Autodesk Fusion 360 part; units mm, degrees
sketch "baseplate" plane through (0, 0, 0) normal (0, 1, 0) x (1, 0, 0)
  line L0 (0, 0) -> (80, 0)
  line L1 (80, 0) -> (80, -40)
  line L2 (80, -40) -> (0, -40)
  line L3 (0, -40) -> (0, 0)
  dimension "d1" = 80
  dimension "d2" = 40
sketch "pryamid_base" plane through (0, 0, 0) normal (0, 1, 0) x (1, 0, 0)
  line L0 (5, -35) -> (15, -35)
  line L1 (15, -35) -> (15, -25)
  line L2 (15, -25) -> (5, -25)
  line L3 (5, -25) -> (5, -35)
  line L4 (35, -35) -> (35, -25)
  line L5 (35, -25) -> (25, -25)
  line L6 (25, -35) -> (35, -35)
  line L7 (25, -25) -> (25, -35)
  line L8 (75, -35) -> (75, -25)
  line L9 (45, -35) -> (55, -35)
  line L10 (55, -25) -> (45, -25)
  line L11 (65, -25) -> (65, -35)
  line L12 (65, -35) -> (75, -35)
  line L13 (55, -35) -> (55, -25)
  line L14 (45, -25) -> (45, -35)
  line L15 (75, -25) -> (65, -25)
  line L16 (35, -5) -> (25, -5)
  line L17 (35, -15) -> (35, -5)
  line L18 (15, -5) -> (5, -5)
  line L19 (25, -5) -> (25, -15)
  line L20 (45, -15) -> (55, -15)
  line L21 (55, -15) -> (55, -5)
  line L22 (5, -5) -> (5, -15)
  line L23 (45, -5) -> (45, -15)
  line L24 (75, -15) -> (75, -5)
  line L25 (65, -5) -> (65, -15)
  line L26 (75, -5) -> (65, -5)
  line L27 (55, -5) -> (45, -5)
  line L28 (65, -15) -> (75, -15)
  line L29 (5, -15) -> (15, -15)
  line L30 (15, -15) -> (15, -5)
  line L31 (25, -15) -> (35, -15)
  dimension "d3" = 10
  dimension "d4" = 10
  dimension "d5" = 10
  dimension "d6" = 10
  dimension "d7" = 10
  dimension "d8" = 10
  dimension "d9" = 10
  dimension "d10" = 10
  dimension "d11" = 10
  dimension "d12" = 10
  dimension "d13" = 10
  dimension "d14" = 10
  dimension "d15" = 10
  dimension "d16" = 10
  dimension "d17" = 10
  dimension "d18" = 10
ref_plane "WorkPlane1" through (0, 4.5, 0) normal (0, 1, 0) x (0, 0, 1)
sketch "pryamid_offsetplane" plane through (0, 4.5, 0) normal (0, 1, 0) x (1, 0, 0)
  line L0 (7.5, -32.5) -> (12.5, -32.5)
  line L1 (12.5, -32.5) -> (12.5, -27.5)
  line L2 (12.5, -27.5) -> (7.5, -27.5)
  line L3 (7.5, -27.5) -> (7.5, -32.5)
  line L4 (27.5, -27.5) -> (27.5, -32.5)
  line L5 (32.5, -32.5) -> (32.5, -27.5)
  line L6 (27.5, -32.5) -> (32.5, -32.5)
  line L7 (32.5, -27.5) -> (27.5, -27.5)
  line L8 (7.5, -27.5) -> (7.5, -32.5)
  line L9 (12.5, -32.5) -> (12.5, -27.5)
  line L10 (7.5, -32.5) -> (12.5, -32.5)
  line L11 (12.5, -27.5) -> (7.5, -27.5)
  line L12 (47.5, -27.5) -> (47.5, -32.5)
  line L13 (52.5, -32.5) -> (52.5, -27.5)
  line L14 (47.5, -32.5) -> (52.5, -32.5)
  line L15 (52.5, -27.5) -> (47.5, -27.5)
  line L16 (67.5, -27.5) -> (67.5, -32.5)
  line L17 (72.5, -32.5) -> (72.5, -27.5)
  line L18 (67.5, -32.5) -> (72.5, -32.5)
  line L19 (72.5, -27.5) -> (67.5, -27.5)
  line L20 (72.5, -12.5) -> (72.5, -7.5)
  line L21 (27.5, -7.5) -> (27.5, -12.5)
  line L22 (12.5, -12.5) -> (12.5, -7.5)
  line L23 (72.5, -7.5) -> (67.5, -7.5)
  line L24 (12.5, -7.5) -> (7.5, -7.5)
  line L25 (52.5, -12.5) -> (52.5, -7.5)
  line L26 (7.5, -7.5) -> (7.5, -12.5)
  line L27 (7.5, -12.5) -> (12.5, -12.5)
  line L28 (47.5, -12.5) -> (52.5, -12.5)
  line L29 (67.5, -7.5) -> (67.5, -12.5)
  line L30 (47.5, -7.5) -> (47.5, -12.5)
  line L31 (67.5, -12.5) -> (72.5, -12.5)
  line L32 (32.5, -7.5) -> (27.5, -7.5)
  line L33 (52.5, -7.5) -> (47.5, -7.5)
  line L34 (27.5, -12.5) -> (32.5, -12.5)
  line L35 (12.5, -7.5) -> (7.5, -7.5)
  line L36 (32.5, -12.5) -> (32.5, -7.5)
  line L37 (12.5, -12.5) -> (12.5, -7.5)
  line L38 (7.5, -12.5) -> (12.5, -12.5)
  line L39 (7.5, -7.5) -> (7.5, -12.5)
extrude "Extrude1" add sketch "baseplate" against normal blind 5
loft "Loft1" add profiles "pryamid_base", "pryamid_offsetplane" section 1 contours L0 L1 L2 L3 section 2 contours L0 L1 L2 L3 L8 L9 L10 L11
loft "Loft2" add profiles "pryamid_base", "pryamid_offsetplane" section 1 contours L4 L5 L6 L7 section 2 contours L4 L5 L6 L7
loft "Loft3" add profiles "pryamid_base", "pryamid_offsetplane" section 1 contours L9 L10 L13 L14 section 2 contours L12 L13 L14 L15
loft "Loft4" add profiles "pryamid_base", "pryamid_offsetplane" section 1 contours L8 L11 L12 L15 section 2 contours L16 L17 L18 L19
loft "Loft5" add profiles "pryamid_base", "pryamid_offsetplane" section 1 contours L24 L25 L26 L28 section 2 contours L20 L23 L29 L31
loft "Loft6" add profiles "pryamid_base", "pryamid_offsetplane" section 1 contours L20 L21 L23 L27 section 2 contours L25 L28 L30 L33
loft "Loft7" add profiles "pryamid_base", "pryamid_offsetplane" section 1 contours L16 L17 L19 L31 section 2 contours L21 L32 L34 L36
loft "Loft8" add profiles "pryamid_base", "pryamid_offsetplane" section 1 contours L18 L22 L29 L30 section 2 contours L22 L24 L26 L27 L35 L37 L38 L39
sketch "sidewall" plane through (0, 0, 0) normal (0, 1, 0) x (1, 0, 0)
  line L0 (0, 0) -> (-8, 0)
  line L1 (-8, 0) -> (-8, -40)
  line L2 (-8, -40) -> (0, -40)
  line L3 (0, -40) -> (0, 0)
  dimension "d22" = 8
extrude "Extrude2" add sketch "sidewall" along normal blind 0 and the other way blind 5
sketch "sidemount" plane through (0, 0, 0) normal (0, 1, 0) x (1, 0, 0)
  line L0 (80, 0) -> (88, 0)
  line L1 (88, 0) -> (88, -40)
  line L2 (88, -40) -> (80, -40)
  line L3 (80, -40) -> (80, 0)
extrude "Extrude3" add sketch "sidemount" against normal blind 5
sketch "holes" plane through (0, -5, 0) normal (0, -1, 0) x (1, 0, 0)
  line L0 (88, 40) -> (-8, 40)
  line L1 (-8, 40) -> (-8, 0)
  line L2 (-8, 0) -> (88, 0)
  line L3 (88, 0) -> (88, 40)
  line L4 (-8, 0) -> (-4, 0)
  line L5 (-8, 6) -> (-8, 0)
  line L6 (-4, 40) -> (-8, 40)
  line L7 (-8, 40) -> (-8, 34)
  circle A0 centre (-4, 34) radius 2
  circle A1 centre (-4, 6) radius 2
  circle A2 centre (-4, 34) radius 3.4
  circle A3 centre (-4, 6) radius 3.4
  dimension "d29" = 6
  dimension "d30" = 4
  dimension "d31" = 4
  dimension "d32" = 6.8
  dimension "d33" = 6.8
extrude "Extrude4" cut sketch "holes" against normal blind 51 contours A0 | A1
sketch "Sketch7" plane through (0, -5, 0) normal (0, -1, 0) x (1, 0, 0)
  circle A0 centre (84, 34) radius 2
  circle A1 centre (84, 6) radius 2
  circle A2 centre (84, 34) radius 3.4
  circle A3 centre (84, 6) radius 3.4
  dimension "d42" = 4
  dimension "d43" = 4
  dimension "d44" = 6.8
  dimension "d45" = 6.8
extrude "Extrude6" cut sketch "Sketch7" against normal blind 16 contours A0 | A1
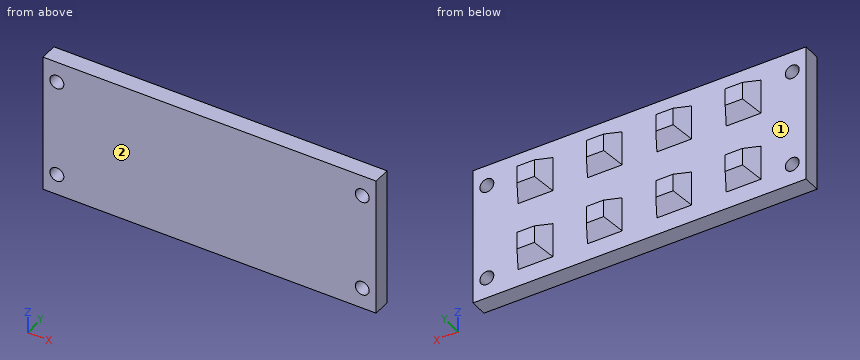
For this review, take the finished solid that the model builds, in its own axes (mm). Face numbers are marked on the shaded views. Round coordinates to 2 decimals unless told otherwise and drop trailing zeros. Order: outer loops, then holes, each group sorted by start corner. A loop starts at its lowest first (then second) coordinate and runs counter-clockwise, first axis right, second up.
Q1. We need section A-A, the plane x = 84. Give the boundary of the cut face in (y, z).
Findings below:
outline: (-5, 0) - (0, 0) - (0, 4) - (-5, 4) - close; (-5, 8) - (0, 8) - (0, 32) - (-5, 32) - close; (-5, 36) - (0, 36) - (0, 40) - (-5, 40) - close
Q2. Wall thickness on line 1 (Z direction, x = 84, y = -1.75); line 2 (X direction, y = -0.75, z = 5.5); line 3 (X direction, y = 3.25, z = 7.5): over which ranges is each line inside the solid? List them lowest first.
Findings below:
line 1: z = 0 to 4, 8 to 32, 36 to 40
line 2: x = -8 to -5.94, -2.06 to 82.06, 85.94 to 88
line 3: x = 6.81 to 13.19, 26.81 to 33.19, 46.81 to 53.19, 66.81 to 73.19
Q3. Insertion check: P1, Ø10, axis at x = 59.5, z = 14.5, coming from the +Y side; P2, Ø6.5, axis at x = -4, z = 6, coming from the +Y side. Each pin has a flat end and moves straight along its axis. Give the tip position at first contact, or say it passes through.
Findings below:
P1: stops at y = 0.9
P2: stops at y = 0
Q4. We need section B-B, the plane y = 1.75. State how many separate pieces and enclosed holes the cut face has, plus the area to 3 significant figures.
Findings below:
separate pieces: 8
enclosed holes: 0
area: 519 mm2
Q5. Mouldability with a two-part tool opening along X and no side actions: class the marked faces 1 and 2 as pulls with the +X half, pulls with the -X half, needs draft (parallel to the pull), parting line crosses it, or undercut.
Findings below:
face 1: undercut
face 2: needs draft
Q6. We need section C-C, the plane z = 16. Give the boundary of the cut face in (x, y).
Findings below:
outline: (-8, -5) - (88, -5) - (88, 0) - (-8, 0) - close
